For this review, take the finished solid that the model builds, in its own axes (mm). A direction names the side the tool comes from. Round coordinates to 2 decimals unless told otherwise and drop trailing zeros. Order: outer loops, then holes, each group sorted by start corner. A loop starts at its lowest first (then second) coordinate and runs counter-clockwise, first axis right, second up. Notation, with made-up numbers: M 30.5,52 L 73.5,52 A13 cw 73.5,69 Z; hole C 55,-17 d9. An arc over 180 degrees is marked long. Answer as a JSON object with one key per item and string values.
from build123d import *

# Parameters (mm, degrees)
F_10_32_TAPPED_HOLE2_D           = 4.0386
F_10_32_TAPPED_HOLE2_DEPTH       = 11.176
F_10_32_TAPPED_HOLE2_CBORE_D     = 4.826
F_10_32_TAPPED_HOLE2_CBORE_DEPTH = 9.652
F_10_32_TAPPED_HOLE2_TIP         = 1.213317848
CUT_EXTRUDE1_DEPTH               = 864.378412287
CUT_EXTRUDE1_DEPTH_BACK          = 864.378412287


with BuildPart() as part:
    # Sketch2 one side → Revolve1 (revolve)
    with BuildSketch(Plane(origin=(0, 0, 0), x_dir=(1, 0, 0), z_dir=(0, 1, 0)), mode=Mode.PRIVATE) as revolve1_sk:
        with BuildLine():
            Line((148.49475, 836.728797606), (151.66975, 836.728797606))
            ThreePointArc((151.66975, 836.728797606), (150.08225, 838.316297606), (148.49475, 836.728797606))
        make_face()
        Polygon((135.001, 836.728797606), (154.051, 836.728797606), (154.051, 843.078797606), (139.7635, 843.078797606), (139.7635, 845.999797606), (138.176, 845.999797606), (138.176, 849.428797606), (135.001, 849.428797606), (135.001, 843.078797606), (135.001, 840.697547606), align=None)
        with BuildLine():
            ThreePointArc((151.66975, 836.728797606), (150.08225, 838.316297606), (148.49475, 836.728797606))
            Line((148.49475, 836.728797606), (151.66975, 836.728797606))
        make_face()
        with BuildLine():
            Line((151.66975, 836.728797606), (148.49475, 836.728797606))
            ThreePointArc((148.49475, 836.728797606), (150.08225, 835.141297606), (151.66975, 836.728797606))
        make_face()
    revolve(revolve1_sk.sketch.rotate(Axis((135.001, 0, -836.728797606), (1, 0, 0)), 180), axis=Axis((135.001, 0, -836.728797606), (1, 0, 0)))

    # 10-32 Tapped Hole2
    with Locations(Plane.ZY.offset(-135.001)):
        with Locations((-836.728797606, 0)):
            CounterBoreHole(F_10_32_TAPPED_HOLE2_D / 2, F_10_32_TAPPED_HOLE2_CBORE_D / 2, F_10_32_TAPPED_HOLE2_CBORE_DEPTH, depth=F_10_32_TAPPED_HOLE2_DEPTH)
            with Locations((0, 0, -(F_10_32_TAPPED_HOLE2_DEPTH + F_10_32_TAPPED_HOLE2_TIP / 2))):  # 118° drill point
                Cone(0, F_10_32_TAPPED_HOLE2_D / 2, F_10_32_TAPPED_HOLE2_TIP, mode=Mode.SUBTRACT)

    # Sketch2_3 → Cut-Extrude1 (cut, two sides: drawn at the far end of the back side and taken through both)
    with BuildSketch(Plane(origin=(0, 0, 0), x_dir=(1, 0, 0), z_dir=(0, 1, 0)).offset(-CUT_EXTRUDE1_DEPTH_BACK)):
        with BuildLine():
            ThreePointArc((151.66975, 836.728797606), (150.08225, 838.316297606), (148.49475, 836.728797606))
            Line((148.49475, 836.728797606), (151.66975, 836.728797606))
        make_face()
        with BuildLine():
            Line((151.66975, 836.728797606), (148.49475, 836.728797606))
            ThreePointArc((148.49475, 836.728797606), (150.08225, 835.141297606), (151.66975, 836.728797606))
        make_face()
    extrude(amount=CUT_EXTRUDE1_DEPTH + CUT_EXTRUDE1_DEPTH_BACK, mode=Mode.SUBTRACT)


solid = part.part
1) For L1, parallel to X at y = 6.75, z = -846.25; L2, parallel to X at y = -6.25, z = -843.5; L3, parallel to Z at x = 149, y = 3, list the stretches that pass through material, from the lowest coordinate up.
Geometry check:
{"L1": "x = 135 to 138.18", "L2": "x = 135 to 139.76", "L3": "z = -842.33 to -837.89, -835.57 to -831.13"}
2) Add section D-D on x = 150.5. State the section outline as (y, z) points.
Geometry check:
{"outline": "M -6.16,-838.26 A6.35 ccw 6.16,-838.26 Z; M -6.16,-835.2 L 6.16,-835.2 A6.35 ccw Z"}
3) Mouldability with a two-part tool opening along Z and no side actions: class faces 1 (the flat face through (138.176, 7.5, -831)), 2 (the cylindrical face through (150.426, -0.089, -838.279)), 3 (the cylindrical face through (138.959, 5.641, -844.086)), 4 (the cylindrical face through (145.43, 0.09, -834.71)) as +Z half, -Z half, draft (parallel to the pull), parting line (faces both ways), or undercut.
Geometry check:
{"face 1": "draft", "face 2": "undercut", "face 3": "parting line", "face 4": "undercut"}
4) Add section A-A on y = -8.75. State the section outline as (x, z) points.
Geometry check:
{"outline": "M 135,-845.93 L 138.18,-845.93 L 138.18,-839.79 L 139.76,-839.79 L 139.76,-833.66 L 138.18,-833.66 L 138.18,-827.52 L 135,-827.52 Z"}
5) Machinability: for faces 5 (the cylindrical face through (146.81, 2.43, -830.86)), 6 (the flat face through (154.051, 0, -837)), 7 (the cylindrical face through (139.76, 0.11, -839.14)), which of the approach directions +Z, -Z, +X, -X, +Y, -Y give a long, thin tool a straight path to every point of the face, cutting with its end or side? Answer none if there is none.
Geometry check:
{"face 5": "+X", "face 6": "+Z, -Z, +X, +Y, -Y", "face 7": "-X"}
6) Add section B-B on x = 143. State the section outline as (y, z) points, and give its area (3 significant figures).
Geometry check:
{"outline": "C 0,-836.73 d12.7; hole C 0,-836.73 d4.83", "area": "108 mm²"}
7) Insertion check: P1, Ø4, axis at x = 139.5, y = 7, coming from the +Z side; P2, Ø8, axis at x = 147.5, z = -832.5, coming from the -Y side; P3, Ø1.4, axis at y = 0.5, z = -837.5, coming from the -X side. Each pin has a flat end and moves straight along its axis. Give the tip position at first contact, or say it passes through.
Geometry check:
{"P1": "stops at z = -825.28", "P2": "stops at y = -6.35", "P3": "stops at x = 146.42"}
8) Add section C-C on z = -832.5. State the section outline as (x, y) points, and give its area (3 significant figures).
Geometry check:
{"outline": "M 135,-11.98 L 138.18,-11.98 L 138.18,-8.25 L 139.76,-8.25 L 139.76,-4.74 L 154.05,-4.74 L 154.05,4.74 L 139.76,4.74 L 139.76,8.25 L 138.18,8.25 L 138.18,11.98 L 135,11.98 Z", "area": "238 mm²"}
